Could you check a few things on this model? Use its own coordinates, in mm. A direction names the side the tool comes from. Give positions to 0.01 mm unless a question says otherwise; leave off trailing zeros. Loops run counter-clockwise (first coordinate to the right, second up) from the corner with the lowest first, then second, coordinate; pieces in that order, holes last. Notation, with made-up numbers: M 86.5,30.25 L 130.5,30.25 A20 cw 130.5,60.25 Z; hole C 1.5,-4 d7. An arc over 180 degrees is marked long. Use CSV: the item, a comma, the result in double quotes.
```python
from build123d import *

# Parameters (mm, degrees)
F1_DEPTH = 38.1


with BuildPart() as f1:
    # F0 (on Top) → F1 (new body)
    with BuildSketch(Plane.XY):
        Polygon((0, 25.4), (0, 0), (-25.4, 0), (-25.4, -5.08), (0, -5.08), (0, -30.479991), (5.08, -30.479991), (5.08, -5.079991), (30.470396, -5.079991), (30.48, 0), (5.08, 0), (5.08, 25.4), align=None)
        Polygon((0, -2.54), (2.54, 0), (5.08, -2.539995), (2.54, -5.079995), align=None, mode=Mode.SUBTRACT)
    extrude(amount=F1_DEPTH)


solid = f1.part
```
1. Please list where these lines run through material, in increasing order: line 1 (X direction, y = 11, z = 25); line 2 (Y direction, x = -23, z = 11); line 3 (Y direction, x = 4, z = 23.5).
Outcome:
line 1,"0 to 5.08"
line 2,"-5.08 to 0"
line 3,"-30.48 to -3.62, -1.46 to 25.4"
2. I'm going to push flat-ended pins straight in: pin 1 Ø5 at (y, z) = (7, 25.5) entering from -X; pin 2 Ø12.5 at (x, z) = (22, 10.5) entering from -Y; pin 3 Ø12.5 at (x, z) = (12, 26.5) entering from +Y. Where does each tip first touch, or does it pass through?
Outcome:
pin 1,"x = 0"
pin 2,"y = -5.08"
pin 3,"y = 0"
3. If we mould it in two halves opening along Y, with no side actions, what happens to faces 4 (the face through (0, 13, 19)), 5 (the face through (1.29, -3.83, 18.78)), 6 (the face through (3, 25.4, 19)), 7 (the face through (18, -5.08, 19))? For each: +Y half, -Y half, draft (parallel to the pull), parting line (faces both ways), or undercut.
Outcome:
face 4,"draft"
face 5,"undercut"
face 6,"+Y half"
face 7,"-Y half"
4. Which directions (+Z, -Z, +X, -X, +Y, -Y) give clear straight access to the entire face, cutting with the end or side of a thin tool? Please do faces 1 (the face through (-13, -5.08, 19)), 2 (the face through (5.08, -18, 19)), 3 (the face through (-13, 0, 19)).
Outcome:
face 1,"+Z, -Z, -X, -Y"
face 2,"+Z, -Z, +X, -Y"
face 3,"+Z, -Z, -X, +Y"
5. I want a section at A-A, the plane z = 17. List the corners of the cut face in (x, y) for me.
Outcome:
outline,"M -25.4,-5.08 L 0,-5.08 L 0,-30.48 L 5.08,-30.48 L 5.08,-5.08 L 30.47,-5.08 L 30.48,0 L 5.08,0 L 5.08,25.4 L 0,25.4 L 0,0 L -25.4,0 Z; hole M 0,-2.54 L 2.54,-5.08 L 5.08,-2.54 L 2.54,0 Z"
6. I want a section at B-B, the plane x = 18. List the corners of the cut face in (y, z) for me, then the cut area to 3 significant figures.
Outcome:
outline,"M -5.08,0 L 0,0 L 0,38.1 L -5.08,38.1 Z"
area,"194 mm2"
7. I want a section at C-C, the plane y = -14. List the corners of the cut face in (x, z) for me.
Outcome:
outline,"M 0,0 L 5.08,0 L 5.08,38.1 L 0,38.1 Z"
